from build123d import *

# Parameters (mm, degrees)
SKETCH2_R           = 10
BOSS_EXTRUDE1_DEPTH = 580
SKETCH3_R           = 5
BOSS_EXTRUDE2_DEPTH = 30
CUT_EXTRUDE1_START  = -10
SKETCH8_W           = 8
SKETCH8_H           = 8
CUT_EXTRUDE1_DEPTH  = 40
SKETCH7_R           = 137
BOSS_EXTRUDE7_DEPTH = 10
FILLET1_R           = 5


with BuildPart() as part:
    # Sketch2 → Boss-Extrude1 (new body)
    with BuildSketch(Plane(origin=(0, 0, 0), x_dir=(0, 0, -1), z_dir=(1, 0, 0))):
        Circle(SKETCH2_R)
    extrude(amount=-BOSS_EXTRUDE1_DEPTH)

    # Sketch3 → Boss-Extrude2 (add)
    with BuildSketch(Plane.ZY.offset(580)):
        Circle(SKETCH3_R)
    extrude(amount=BOSS_EXTRUDE2_DEPTH)

    # Sketch8 → Cut-Extrude1 (cut)
    with BuildSketch(Plane.ZY.offset(580).offset(CUT_EXTRUDE1_START)):
        with Locations((0, 10)):
            Rectangle(SKETCH8_W, SKETCH8_H)
    extrude(amount=-CUT_EXTRUDE1_DEPTH, mode=Mode.SUBTRACT)

    # Sketch7 → Boss-Extrude7 (add)
    with BuildSketch(Plane(origin=(0, 0, 0), x_dir=(0, 0, -1), z_dir=(1, 0, 0))):
        Circle(SKETCH7_R)
        with BuildLine():
            Line((-10, 23.094010768), (-70.845389143, 58.223112568))
            ThreePointArc((-70.845389143, 58.223112568), (-80.785784301, 74.000688066), (-73.390830204, 91.119624901))
            ThreePointArc((-73.390830204, 91.119624901), (0, 117), (73.390830204, 91.119624901))
            ThreePointArc((73.390830204, 91.119624901), (80.785784301, 74.000688066), (70.845389143, 58.223112568))
            Line((70.845389143, 58.223112568), (10, 23.094010768))
            ThreePointArc((10, 23.094010768), (0, 20.414518843), (-10, 23.094010768))
        make_face(mode=Mode.SUBTRACT)
        with BuildLine():
            Line((-15, -20.207259422), (-15, -90.465463023))
            ThreePointArc((-15, -90.465463023), (-23.693583612, -106.962885502), (-42.216494845, -109.118135811))
            ThreePointArc((-42.216494845, -109.118135811), (-101.324972243, -58.5), (-115.607325049, 17.998510911))
            ThreePointArc((-115.607325049, 17.998510911), (-104.479367913, 32.962197437), (-85.845389143, 32.242350455))
            Line((-85.845389143, 32.242350455), (-25, -2.886751346))
            ThreePointArc((-25, -2.886751346), (-17.679491924, -10.207259422), (-15, -20.207259422))
        make_face(mode=Mode.SUBTRACT)
        with BuildLine():
            Line((25, -2.886751346), (85.845389143, 32.242350455))
            ThreePointArc((85.845389143, 32.242350455), (104.479367913, 32.962197437), (115.607325049, 17.998510911))
            ThreePointArc((115.607325049, 17.998510911), (101.324972243, -58.5), (42.216494845, -109.118135811))
            ThreePointArc((42.216494845, -109.118135811), (23.693583612, -106.962885502), (15, -90.465463023))
            Line((15, -90.465463023), (15, -20.207259422))
            ThreePointArc((15, -20.207259422), (17.679491924, -10.207259422), (25, -2.886751346))
        make_face(mode=Mode.SUBTRACT)
    extrude(amount=-BOSS_EXTRUDE7_DEPTH)

    # Fillet1
    fillet1_edges = [part.edges().sort_by_distance(p)[0] for p in [
        (0, 0, 137),
    ]]
    fillet(fillet1_edges, radius=FILLET1_R)


solid = part.part
CAD build for the part. Positions are in the model's coordinates, mm. A direction names the side the tool comes from. Round coordinates to 2 decimals unless told otherwise and drop trailing zeros. Write each loop counter-clockwise with the first axis right and the second up, starting at its lowest first coordinate (ties: lowest second). Pieces come first, ordered by that corner, then holes.
(1) 3-axis set-ups, long thin cutter, end or side, ignore diameter. For faces 1 (the face through (-4.93, 32.843, 104.724)), 2 (the face through (0, 2, 2)), 3 (the face through (-580, -2, 5)): which of +Z, -Z, +X, -X, +Y, -Y reach the whole face in a straight line?
(2) Probe line 1 along X through (y, z) = (6, -39); line 2 along Z through (x, y) = (-523.5, -9). List the from-to ranges inside material, lowest first.
(3) Slice it at A-A, the plane x = -325. Write the cut outline in (y, z).
(4) Slice it at B-B, the plane y = -74.5. Count the separate pieces of the cut face and the enclosed holes in it, and give its area (3 significant figures).
(5) Slice it at C-C, the plane x = -563. Write the cut outline in (y, z).
(6) Drop flat-ended pins along their axis: P1, Ø8, axis at x = -303.5, z = 9.5, coming from the -Y side; P2, Ø11, axis at x = -3, y = -58.5, coming from the -Z side; P3, Ø2, axis at y = 7, z = 1, coming from the -X side. Give the stop position or say it passes through.
(7) Mould opens along Y. For faces 4 (the face through (-4.93, 40.904, -40.849)), 5 (the face through (-7.465, 41.151, -130.674)), 6 (the face through (-10, 2, -29)) say: pulls with the +Y half, pulls with the -Y half, needs draft (parallel to the pull), parting line crosses it, or undercut.
From the geometry:
1. face 1: +X, -X
1. face 2: +Z, -Z, +X, +Y, -Y
1. face 3: -X
2. line 1: x = -10 to 0
2. line 2: z = -4.36 to 4.36
3. outline: circle Ø20 at (0, 0)
4. separate pieces: 3
4. enclosed holes: 0
4. area: 782 mm2
5. outline: (6, -4) - (6, 4) - (9.17, 4) arc R10 ccw (long way) to (9.17, -4) - close
6. P1: stops at y = -8.35
6. P2: stops at z = -126.22
6. P3: stops at x = -580
7. face 4: undercut
7. face 5: parting line crosses it
7. face 6: needs draft
